Part print with two shaded views. Sizes in mm from the minimum x, y, z corner. A direction names the side the tool comes from. Round coordinates to 2 decimals unless told otherwise and drop trailing zeros. Order: outer loops, then holes, each group sorted by start corner. A loop starts at its lowest first (then second) coordinate and runs counter-clockwise, first axis right, second up. Notation, with made-up numbers: M 17,-34 L 56,-34 A35 cw 56,2 Z; hole C 43,49.5 d6. An arc over 180 degrees is marked long. Return JSON: item names as keys, results as strings. Group by question number.
Item 1: Probe line 1 along Y through (x, z) = (2.5, 29.1); line 2 along X through (y, z) = (5, 27.75); line 3 along Y through (x, z) = (2, 29) (1 decimal). List the from-to ranges inside material, lowest first.
Item 2: Slice it at A-A on x = 2.5. Write the cut outline in (y, z).
Item 3: Pin check, flat tips, straight feed: pin 1 Ø5 at (y, z) = (9.5, 35) entering from +X; pin 2 Ø4 at (x, y) = (50.5, 5) entering from +Z; pin 3 Ø3 at (y, z) = (11.5, 27) entering from -X; pin 4 Ø2 at (x, y) = (25.5, 9.5) entering from +Z. Stop position of each tip, or through.
Item 4: Slice it at B-B on z = 28.5. Write the cut outline in (x, y).
Item 5: Which spindle directions (+Z, -Z, +X, -X, +Y, -Y) get a long thin tool onto all of the face, cutting with end or side? Do the marked faces 1, 2 and 3. Say none if no direction does.
Item 6: Slice it at C-C on z = 35. Write the cut outline in (x, y) (1 decimal).
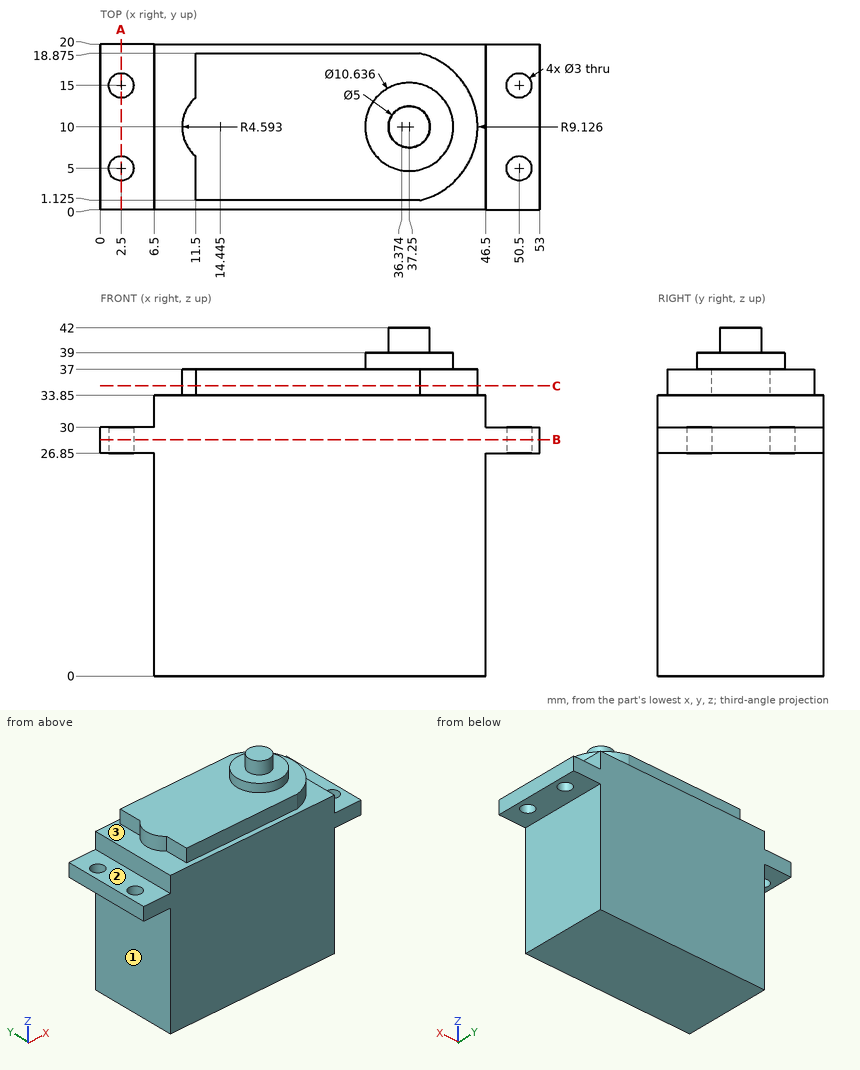
Output values:
{
 "1": {"line 1": "0 to 3.5, 6.5 to 13.5, 16.5 to 20", "line 2": "0 to 1, 4 to 49, 52 to 53", "line 3": "0 to 3.6, 6.4 to 13.6, 16.4 to 20"},
 "2": {"outline": "M 0,26.85 L 3.5,26.85 L 3.5,30 L 0,30 Z; M 6.5,26.85 L 13.5,26.85 L 13.5,30 L 6.5,30 Z; M 16.5,26.85 L 20,26.85 L 20,30 L 16.5,30 Z"},
 "3": {"pin 1": "x = 46.5", "pin 2": "z = 30", "pin 3": "x = 0", "pin 4": "z = 37"},
 "4": {"outline": "M 0,0 L 53,0 L 53,20 L 0,20 Z; hole C 2.5,5 d3; hole C 2.5,15 d3; hole C 50.5,5 d3; hole C 50.5,15 d3"},
 "5": {"face 1": "-Z, -X, +Y, -Y", "face 2": "+Z, -X, +Y, -Y", "face 3": "+Z"},
 "6": {"outline": "M 11.5,1.1 L 38.5,1.1 A9.1 ccw 38.5,18.9 L 11.5,18.9 L 11.5,13.5 A4.6 ccw 11.5,6.5 Z"}
}
